```python
from build123d import *

# Parameters (mm, degrees)
SCHIZZO1_W                   = 375
SCHIZZO1_H                   = 375
ESTRUSIONE_ESTRUSIONE1_DEPTH = 5
TAGLIO_ESTRUSIONE1_REACH     = 267.212
SCHIZZO2_R                   = 62.5
FORO_PER_VITE_M3_4_D         = 3.4
RIPETIZIONECIRCOLARE1_COUNT  = 3
FORO_PER_VITE_M3_2_D         = 3.4
RIPETIZIONECIRCOLARE3_COUNT  = 3
FORO_PER_VITE_M3_5_D         = 3.4
RIPETIZIONECIRCOLARE4_COUNT  = 3


with BuildPart() as part:
    # Schizzo1 → Estrusione-Estrusione1 (new body)
    with BuildSketch(Plane.XY):
        Rectangle(SCHIZZO1_W, SCHIZZO1_H)
    extrude(amount=ESTRUSIONE_ESTRUSIONE1_DEPTH)

    # Schizzo2 → Taglio-Estrusione1 (cut, up to next)
    with BuildSketch(Plane.XY.offset(5), mode=Mode.PRIVATE) as taglio_estrusione1_sk1:
        Circle(SCHIZZO2_R)
    taglio_estrusione1_tool1 = extrude(taglio_estrusione1_sk1.sketch, amount=-TAGLIO_ESTRUSIONE1_REACH, mode=Mode.PRIVATE) & part.part
    add(taglio_estrusione1_tool1.solids().sort_by_distance((0, 0, 5))[0], mode=Mode.SUBTRACT)

    # Foro per Vite M3-4 (through all)
    with Locations(Plane.XY.offset(5)):
        with Locations((-26.307698917, -149.198374581), (26.307698917, -149.198374581)):
            foro_per_vite_m3_4 = Hole(FORO_PER_VITE_M3_4_D / 2)

    # RipetizioneCircolare1: Foro per Vite M3-4 ×3 about axis
    ripetizionecircolare1_axis = Axis((0, 0, 0), (0, 0, 1))
    for i in range(1, RIPETIZIONECIRCOLARE1_COUNT):
        add(foro_per_vite_m3_4.rotate(ripetizionecircolare1_axis, i * 360 / RIPETIZIONECIRCOLARE1_COUNT), mode=Mode.SUBTRACT)

    # Foro per Vite M3-2 (through all)
    with Locations(Plane.XY.offset(5)):
        with Locations((-25.309490606, -69.537253938)):
            foro_per_vite_m3_2 = Hole(FORO_PER_VITE_M3_2_D / 2)

    # RipetizioneCircolare3: Foro per Vite M3-2 ×3 about axis
    ripetizionecircolare3_axis = Axis((0, 0, 0), (0, 0, 1))
    for i in range(1, RIPETIZIONECIRCOLARE3_COUNT):
        add(foro_per_vite_m3_2.rotate(ripetizionecircolare3_axis, i * 360 / RIPETIZIONECIRCOLARE3_COUNT), mode=Mode.SUBTRACT)

    # Foro per Vite M3-5 (through all)
    with Locations(Plane.XY.offset(5)):
        with Locations((67.638784068, 134.153810568), (82.361215932, 125.653810568)):
            foro_per_vite_m3_5 = Hole(FORO_PER_VITE_M3_5_D / 2)

    # RipetizioneCircolare4: Foro per Vite M3-5 ×3 about axis
    ripetizionecircolare4_axis = Axis((0, 0, 0), (0, 0, 1))
    for i in range(1, RIPETIZIONECIRCOLARE4_COUNT):
        add(foro_per_vite_m3_5.rotate(ripetizionecircolare4_axis, i * 360 / RIPETIZIONECIRCOLARE4_COUNT), mode=Mode.SUBTRACT)


solid = part.part
```
Build history of the part. All positions in model axes, mm. Coordinates: 2 decimals unless noted, no trailing zeros. Order: outer loops, then holes, each group sorted by start corner. A loop starts at its lowest first (then second) coordinate and runs counter-clockwise, first axis right, second up. Notation, with made-up numbers: (71, 84.25) -> (129, 84.25) arc R11 ccw to (129, 92.25) -> close; hole circle Ø5 at (69.25, -1). An arc over 180 degrees is marked (long way). Answer in a Markdown table with one row per item. Add a question column.
Q1. Wall check: line 1 along X through (y, z) = (-149, 2.45); line 2 along Y through (x, z) = (82.5, 4.05); line 3 along Y through (x, z) = (-150, 3.4). Give the ranges that are in metal, low to high. Write a range as [from, to].
Q2. Mould opens along Y. For faces 1 (the face through (-62.44, 2.75, 2.54)), 2 (the face through (-86, 3, 0)) say: +Y half, -Y half, draft (parallel to the pull), parting line (faces both ways), or undercut.
Q3. Band-saw the part on B-B, the plane x = 11.5. List the corners of the cut face in (y, z), then the cut area to 3 significant figures.
Q4. Band-saw the part on A-A, the plane y = 0. List the corners of the cut face in (x, z), then the cut area to 3 significant figures.
Q5. Band-saw the part on C-C, the plane z = 1.55. Give the number of separate pieces and of enclosed holes in the cut face, then the cut area to 3 significant figures.
Answers follow:
| question | item | result |
|---|---|---|
| 1 | line 1 | [-187.5, -28], [-24.62, 24.62], [28, 187.5] |
| 1 | line 2 | [-187.5, -127.35], [-123.96, 123.96], [127.35, 187.5] |
| 1 | line 3 | [-187.5, -10.2], [-6.8, 6.8], [10.2, 187.5] |
| 2 | face 1 | undercut |
| 2 | face 2 | draft |
| 3 | outline | (-187.5, 0) -> (-61.43, 0) -> (-61.43, 5) -> (-187.5, 5) -> close; (61.43, 0) -> (187.5, 0) -> (187.5, 5) -> (61.43, 5) -> close |
| 3 | area | 1,260 mm^2 |
| 4 | outline | (-187.5, 0) -> (-62.5, 0) -> (-62.5, 5) -> (-187.5, 5) -> close; (62.5, 0) -> (187.5, 0) -> (187.5, 5) -> (62.5, 5) -> close |
| 4 | area | 1,250 mm^2 |
| 5 | separate pieces | 1 |
| 5 | enclosed holes | 16 |
| 5 | area | 128,000 mm^2 |
